```python
from build123d import *

# Parameters (mm, degrees)
F1_DEPTH = 50.8
F2_R     = 5.08
F3_R     = 6.35
F4_DEPTH = 45.72


with BuildPart() as f1:
    # F0 (on Front) → F1 (new body)
    with BuildSketch(Plane.XZ):
        Polygon((635, 25.4), (0, 25.4), (-635, 25.4), (-635, 0), (-635, -25.4), (0, -25.4), (635, -25.4), (635, 0), align=None)
    extrude(amount=F1_DEPTH)

    # F2
    f2_edges = [f1.edges().sort_by_distance(p)[0] for p in [
        (0, -50.8, 25.4),
        (0, 0, 25.4),
        (0, -50.8, -25.4),
        (0, 0, -25.4),
    ]]
    fillet(f2_edges, radius=F2_R)

    # F3 (on face) → F4 (cut)
    with BuildSketch(Plane(origin=(0, 0, -25.4), x_dir=(1, 0, 0), z_dir=(0, 0, -1))):
        with Locations((279.4, 25.4)):
            Circle(F3_R)
        with Locations((609.6, 25.4)):
            Circle(F3_R)
        with Locations((-279.4, 25.4)):
            Circle(F3_R)
        with Locations((-609.6, 25.4)):
            Circle(F3_R)
    extrude(amount=-F4_DEPTH, mode=Mode.SUBTRACT)


solid = f1.part
```
Can you work these out from the model? Positions are in its coordinate system, mm. Coordinates: 2 decimals unless noted, no trailing zeros. Put each result on its own line as item: value. Start each with the question number.
(1) We'd pull the mould along X, two halves only. Please class faces 1 (the face through (635, -25, 0)), 2 (the face through (-635, -25, 0)), 3 (the face through (9, -25, 25.4)): +X half, -X half, draft (parallel to the pull), parting line (faces both ways), or undercut.
(2) Will this pin go through, and if not, where does the flat tip stop? pin 1 Ø7.5 at (x, y) = (-279.4, -25.4) entering from -Z.
(3) I need wall thicknesses on probe 1 along X at (y, z) = (-25.4, 7.5); probe 2 along Y at (x, z) = (279.4, -3.5); probe 3 along X at (y, z) = (-22.5, -0.5). Which ranges of each line are inside material? Lowest first, please.
Worked answers:
1. face 1: +X half
1. face 2: -X half
1. face 3: draft
2. pin 1: stops at z = 20.32
3. probe 1: x = -635 to -615.95, -603.25 to -285.75, -273.05 to 273.05, 285.75 to 603.25, 615.95 to 635
3. probe 2: y = -50.8 to -31.75, -19.05 to 0
3. probe 3: x = -635 to -615.25, -603.95 to -285.05, -273.75 to 273.75, 285.05 to 603.95, 615.25 to 635
